Source: CAD feature listing. Evaluate the final solid. Frame: model axes, mm. A direction names the side the tool comes from. Coordinates: 2 decimals unless noted, no trailing zeros. Write each loop counter-clockwise with the first axis right and the second up, starting at its lowest first coordinate (ties: lowest second). Pieces come first, ordered by that corner, then holes. Notation, with made-up numbers: (-15.5, -21.5) -> (4.5, -21.5) arc R11 ccw to (4.5, -1.5) -> close; hole circle Ø2 at (-18, -11.75). An arc over 180 degrees is marked (long way). One line per item, written item: value. Start each with the question number.
1. Line query: line 1 (X direction, y = 3.25, z = -5.5); line 2 (Z direction, x = 103, y = 3); line 3 (X direction, y = 0.5, z = -8). Output: solid intervals per line, ascending.
2. Section query D-D, the plane z = -42.5. Output: boundary loops of the cut face in (x, y), and give its area (3 significant figures).
3. Section query A-A, the plane y = 4.75. Output: boundary loops of the cut face in (x, z) (3 decimals), and give its area (3 significant figures).
4. Section query B-B, the plane x = 52. Output: boundary loops of the cut face in (y, z), and give its area (3 significant figures).
5. Section query C-C, the plane x = 27. Output: boundary loops of the cut face in (y, z), and give its area (3 significant figures).
6. Mould query, pull axis Z, two halves, no side actions, for faces 1 (the cylindrical face through (8.35, 3.219, -3.966)), 2 (the cylindrical face through (1.8, 3.2, -98.7)), 3 (the flat face through (31, 6.35, -31)). Classes: released by +Z, released by -Z, zero draft, split by the parting line, or undercut.
7. First-contact query: P1, Ø2, axis at y = 5.5, z = -50, coming from the +X side. Flat tip, straight axial feed; report the tip coordinate or a pass-through.
8. Access query for faces 4 (the flat face through (0, 3, -49)), 5 (the flat face through (86, 3, -11.43)). Directions: +Z, -Z, +X, -X, +Y, -Y. A direction counts if a zero-diameter tool reaches every point of the face in a straight line with its end or side. Return the directions, or none.
from build123d import *

# Parameters (mm, degrees)
BOSS_EXTRUDE1_DEPTH = 6.35
FILLET1_R           = 2.54
SKETCH3_R           = 3.81
SKETCH3_R_2         = 3.175
CUT_EXTRUDE1_DEPTH  = 118.627520719
SKETCH7_W           = 11.43
SKETCH7_H           = 6.35
BOSS_EXTRUDE3_DEPTH = 56.642
SKETCH8_W           = 0.889
SKETCH8_H           = 6.35
BOSS_EXTRUDE4_DEPTH = 1.27
FILLET2_R           = 2.54


with BuildPart() as part:
    # Sketch1 → Boss-Extrude1 (new body)
    with BuildSketch(Plane(origin=(0, 0, 0), x_dir=(1, 0, 0), z_dir=(0, 1, 0))):
        Polygon((0, 0), (0, 105.41), (63.5, 0), align=None)
    extrude(amount=BOSS_EXTRUDE1_DEPTH)

    # Fillet1
    fillet1_edges = [part.edges().sort_by_distance(p)[0] for p in [
        (0, 3.175, 0),
        (0, 3.175, -105.41),
    ]]
    fillet(fillet1_edges, radius=FILLET1_R)

    # Sketch3 → Cut-Extrude1 (cut, through all)
    with BuildSketch(Plane(origin=(0, 6.35, 0), x_dir=(1, 0, 0), z_dir=(0, 1, 0))):
        with Locations(Location((5.67299463, 83.963748496, 0), (0, 0, 270))):
            Circle(SKETCH3_R)
        with Locations(Location((5.67299463, 5.67299463, 0), (0, 0, 270))):
            Circle(SKETCH3_R_2)
        with Locations(Location((53.460687214, 5.67299463, 0), (0, 0, 270))):
            Circle(SKETCH3_R_2)
    extrude(amount=-CUT_EXTRUDE1_DEPTH, mode=Mode.SUBTRACT)

    # Sketch7 → Boss-Extrude3 (add)
    with BuildSketch(Plane(origin=(57.15, 0, 0), x_dir=(0, 0, -1), z_dir=(1, 0, 0))):
        with Locations((5.715, 3.175)):
            Rectangle(SKETCH7_W, SKETCH7_H)
    extrude(amount=BOSS_EXTRUDE3_DEPTH)

    # Sketch8 → Boss-Extrude4 (add)
    with BuildSketch(Plane(origin=(57.15, 0, 0), x_dir=(0, 0, -1), z_dir=(1, 0, 0))):
        with Locations((10.9855, 3.175)):
            Rectangle(SKETCH8_W, SKETCH8_H)
    extrude(amount=-BOSS_EXTRUDE4_DEPTH)

    # Fillet2
    fillet2_edges = [part.edges().sort_by_distance(p)[0] for p in [
        (56.614457831, 3.175, -11.43),
    ]]
    fillet(fillet2_edges, radius=FILLET2_R)


solid = part.part
Computed values:
1. line 1: x = 0 to 2.5, 8.84 to 50.29, 56.63 to 113.79
1. line 2: z = -11.43 to 0
1. line 3: x = 0 to 3.51, 7.83 to 51.3, 55.62 to 113.79
2. outline: (0, 0) -> (37.9, 0) -> (37.9, 6.35) -> (0, 6.35) -> close
2. area: 241 mm²
3. outline: (0, -96.271) arc R2.54 ccw to (4.716, -97.582) -> (55.874, -12.659) arc R2.54 cw to (58.05, -11.43) -> (113.792, -11.43) -> (113.792, 0) -> (2.54, 0) arc R2.54 ccw to (0, -2.54) -> close; hole circle Ø7.62 at (5.673, -83.964); hole circle Ø6.35 at (5.673, -5.673); hole circle Ø6.35 at (53.461, -5.673)
3. area: 3,840 mm²
4. outline: (0, -19.09) -> (6.35, -19.09) -> (6.35, -8.49) -> (0, -8.49) -> close; (0, -2.85) -> (6.35, -2.85) -> (6.35, 0) -> (0, 0) -> close
4. area: 85.4 mm²
5. outline: (0, -60.59) -> (6.35, -60.59) -> (6.35, 0) -> (0, 0) -> close
5. area: 385 mm²
6. face 1: undercut
6. face 2: released by -Z
6. face 3: zero draft
7. P1: stops at x = 33.98
8. face 4: +Z, -Z, -X, +Y, -Y
8. face 5: -Z, +X, +Y, -Y
